```python
from build123d import *

# Parameters (mm, degrees)
ESBO_O1_W                = 18
ESBO_O1_H                = 25.5
RESSALTO_EXTRUS_O1_DEPTH = 0.45
ESBO_O2_R                = 0.35
CORTE_EXTRUS_O1_DEPTH    = 16.632418239
ESBO_O3_R                = 0.35
CORTE_EXTRUS_O2_DEPTH    = 16.632418239


with BuildPart() as part:
    # Esboço1 → Ressalto-extrusão1 (new, symmetric)
    with BuildSketch(Plane.XY):
        Rectangle(ESBO_O1_W, ESBO_O1_H)
    extrude(amount=RESSALTO_EXTRUS_O1_DEPTH, both=True)

    # Esboço2 → Corte-extrusão1 (cut, through all)
    with BuildSketch(Plane.XY.offset(0.45)):
        with Locations((-5.72, -12.75)):
            Circle(ESBO_O2_R)
        with Locations((-4.45, -12.75)):
            Circle(ESBO_O2_R)
        with Locations((-3.18, -12.75)):
            Circle(ESBO_O2_R)
        with Locations((-1.91, -12.75)):
            Circle(ESBO_O2_R)
        with Locations((-0.64, -12.75)):
            Circle(ESBO_O2_R)
        with Locations((0.63, -12.75)):
            Circle(ESBO_O2_R)
        with Locations((1.9, -12.75)):
            Circle(ESBO_O2_R)
        with Locations((3.17, -12.75)):
            Circle(ESBO_O2_R)
        with Locations((4.44, -12.75)):
            Circle(ESBO_O2_R)
        with Locations((5.71, -12.75)):
            Circle(ESBO_O2_R)
    extrude(amount=-CORTE_EXTRUS_O1_DEPTH, mode=Mode.SUBTRACT)

    # Esboço3 → Corte-extrusão2 (cut, through all)
    with BuildSketch(Plane.XY.offset(0.45)):
        with Locations((-9, -11.25)):
            Circle(ESBO_O3_R)
        with Locations((-9, -9.98)):
            Circle(ESBO_O3_R)
        with Locations((-9, -8.71)):
            Circle(ESBO_O3_R)
        with Locations((-9, -7.44)):
            Circle(ESBO_O3_R)
        with Locations((-9, -6.17)):
            Circle(ESBO_O3_R)
        with Locations((-9, -4.9)):
            Circle(ESBO_O3_R)
        with Locations((-9, -3.63)):
            Circle(ESBO_O3_R)
        with Locations((-9, -2.36)):
            Circle(ESBO_O3_R)
        with Locations((-9, -1.09)):
            Circle(ESBO_O3_R)
        with Locations((-9, 0.18)):
            Circle(ESBO_O3_R)
        with Locations((-9, 1.45)):
            Circle(ESBO_O3_R)
        with Locations((-9, 2.72)):
            Circle(ESBO_O3_R)
        with Locations((-9, 3.99)):
            Circle(ESBO_O3_R)
        with Locations((9, 3.99)):
            Circle(ESBO_O3_R)
        with Locations((9, 2.72)):
            Circle(ESBO_O3_R)
        with Locations((9, 1.45)):
            Circle(ESBO_O3_R)
        with Locations((9, 0.18)):
            Circle(ESBO_O3_R)
        with Locations((9, -1.09)):
            Circle(ESBO_O3_R)
        with Locations((9, -2.36)):
            Circle(ESBO_O3_R)
        with Locations((9, -3.63)):
            Circle(ESBO_O3_R)
        with Locations((9, -4.9)):
            Circle(ESBO_O3_R)
        with Locations((9, -6.17)):
            Circle(ESBO_O3_R)
        with Locations((9, -7.44)):
            Circle(ESBO_O3_R)
        with Locations((9, -8.71)):
            Circle(ESBO_O3_R)
        with Locations((9, -9.98)):
            Circle(ESBO_O3_R)
        with Locations((9, -11.25)):
            Circle(ESBO_O3_R)
    extrude(amount=-CORTE_EXTRUS_O2_DEPTH, mode=Mode.SUBTRACT)


solid = part.part
```
Design review of the part built by this model. Coordinates are the model's own, in mm. Coordinates: 2 decimals unless noted, no trailing zeros. Order: outer loops, then holes, each group sorted by start corner. A loop starts at its lowest first (then second) coordinate and runs counter-clockwise, first axis right, second up.
1) Take a section at A-A, the plane y = -9.98. Give the boundary of the cut face in (x, z), and give its area (3 significant figures).
2) Wall thickness on line 1 along Y through (x, z) = (-3.25, 0.35); line 2 along X through (y, z) = (2.5, 0.35); line 3 along X through (y, z) = (-9, 0.3): over which ranges is each line inside the solid? List them lowest first.
Returned:
1. outline: (-8.65, -0.45) - (8.65, -0.45) - (8.65, 0.45) - (-8.65, 0.45) - close
1. area: 15.6 mm2
2. line 1: y = -12.41 to 12.75
2. line 2: x = -8.73 to 8.73
2. line 3: x = -8.8 to 8.8
